from build123d import *

# Parameters (mm, degrees)
F0_R     = 1.651
F0_W     = 83.9253333333
F0_H     = 2.54
F0_W_2   = 0.7576921484
F0_H_2   = 0.9999891111
F1_DEPTH = 25.4


with BuildPart() as f1:
    # F0 (on Top) → F1 (new body)
    with BuildSketch(Plane.XY):
        Polygon((-45.2646666667, -11.43), (-49.8366666667, -11.43), (-49.8366666667, -19.05), (49.8366666667, -19.05), (49.8366666667, -11.43), (45.2646666667, -11.43), (41.9626666667, -11.43), (-41.9626666667, -11.43), align=None)
        with Locations((-47.5506666667, -15.0114614516)):
            Circle(F0_R, mode=Mode.SUBTRACT)
        with Locations((0.0100299507, -15.2482278645)):
            Circle(F0_R, mode=Mode.SUBTRACT)
        with Locations((47.5506666667, -15.0114614516)):
            Circle(F0_R, mode=Mode.SUBTRACT)
        with BuildLine():
            Line((-49.8366666667, -19.05), (-49.8366666667, -11.43))
            Line((-49.8366666667, -11.43), (-49.8366666667, -5.0728137152))
            ThreePointArc((-49.8366666667, -5.0728137152), (-51.4876666667, -3.4218137152), (-49.8366666667, -1.7708137152))
            Line((-49.8366666667, -1.7708137152), (-49.8366666667, 1.778))
            Line((-49.8366666667, 1.778), (-54.9166666667, 1.778))
            Line((-54.9166666667, 1.778), (-54.9166666667, -19.05301027))
            Line((-54.9166666667, -19.05301027), (-49.8366666667, -19.05301027))
            Line((-49.8366666667, -19.05301027), (-49.8366666667, -19.05))
        make_face()
        Polygon((-45.2646666667, -0.9999891111), (-45.2646666667, -11.43), (-41.9626666667, -11.43), (-41.9626666667, -8.89), (-41.9626666667, -0.9999891111), (-44.5069745183, -0.9999891111), align=None)
        with Locations((0, -10.16)):
            Rectangle(F0_W, F0_H)
        with Locations((-44.8858205925, -0.4999945555)):
            Rectangle(F0_W_2, F0_H_2)
        with BuildLine():
            Line((49.8366666667, -11.43), (49.8366666667, -19.05))
            Line((49.8366666667, -19.05), (49.8366666667, -19.05301027))
            Line((49.8366666667, -19.05301027), (54.9166666667, -19.05301027))
            Line((54.9166666667, -19.05301027), (54.9166666667, 1.778))
            Line((54.9166666667, 1.778), (49.8366666667, 1.778))
            Line((49.8366666667, 1.778), (49.8366666667, -1.7708137152))
            ThreePointArc((49.8366666667, -1.7708137152), (51.0040999624, -2.2543804195), (51.4876666667, -3.4218137152))
            ThreePointArc((51.4876666667, -3.4218137152), (51.0040999624, -4.589247011), (49.8366666667, -5.0728137152))
            Line((49.8366666667, -5.0728137152), (49.8366666667, -11.43))
        make_face()
        Polygon((41.9626666667, -8.89), (41.9626666667, -11.43), (45.2646666667, -11.43), (45.2646666667, -0.9999891111), (44.5069745183, -0.9999891111), (41.9626666667, -0.9999891111), align=None)
        Polygon((-45.2646666667, 1.778), (-45.2646666667, 0), (-44.5069745183, 0), (-41.94509238, 0), (-45.2646666667, 3.81), align=None)
        with BuildLine():
            Line((-54.9166666667, 1.778), (-49.8366666667, 1.778))
            Line((-49.8366666667, 1.778), (-45.2646666667, 1.778))
            Line((-45.2646666667, 1.778), (-45.2646666667, 3.81))
            Line((-45.2646666667, 3.81), (-52.8846666667, 3.81))
            ThreePointArc((-52.8846666667, 3.81), (-54.321507646, 3.2148409794), (-54.9166666667, 1.778))
        make_face()
        with Locations((44.8858205925, -0.4999945555)):
            Rectangle(F0_W_2, F0_H_2)
        with BuildLine():
            Line((49.8366666667, 1.778), (54.9166666667, 1.778))
            ThreePointArc((54.9166666667, 1.778), (54.321507646, 3.2148409794), (52.8846666667, 3.81))
            Line((52.8846666667, 3.81), (47.8046666667, 3.81))
            Line((47.8046666667, 3.81), (45.2646666667, 3.81))
            Line((45.2646666667, 3.81), (45.2646666667, 1.778))
            Line((45.2646666667, 1.778), (49.8366666667, 1.778))
        make_face()
        Polygon((44.5069745183, 0), (45.2646666667, 0), (45.2646666667, 1.778), (45.2646666667, 3.81), (41.94509238, 0), align=None)
        with BuildLine():
            Line((-49.8366666667, -5.0728137152), (-49.8366666667, -11.43))
            Line((-49.8366666667, -11.43), (-45.2646666667, -11.43))
            Line((-45.2646666667, -11.43), (-45.2646666667, -0.9999891111))
            Line((-45.2646666667, -0.9999891111), (-45.2646666667, 0))
            Line((-45.2646666667, 0), (-45.2646666667, 1.778))
            Line((-45.2646666667, 1.778), (-49.8366666667, 1.778))
            Line((-49.8366666667, 1.778), (-49.8366666667, -1.7708137152))
            ThreePointArc((-49.8366666667, -1.7708137152), (-48.6692333709, -2.2543804195), (-48.1856666667, -3.4218137152))
            ThreePointArc((-48.1856666667, -3.4218137152), (-48.6692333709, -4.589247011), (-49.8366666667, -5.0728137152))
        make_face()
        with BuildLine():
            Line((45.2646666667, -11.43), (49.8366666667, -11.43))
            Line((49.8366666667, -11.43), (49.8366666667, -5.0728137152))
            ThreePointArc((49.8366666667, -5.0728137152), (48.1856666667, -3.4218137152), (49.8366666667, -1.7708137152))
            Line((49.8366666667, -1.7708137152), (49.8366666667, 1.778))
            Line((49.8366666667, 1.778), (45.2646666667, 1.778))
            Line((45.2646666667, 1.778), (45.2646666667, 0))
            Line((45.2646666667, 0), (45.2646666667, -0.9999891111))
            Line((45.2646666667, -0.9999891111), (45.2646666667, -11.43))
        make_face()
    extrude(amount=F1_DEPTH)


solid = f1.part
The listing builds one solid part. Answer for the finished solid, in the listing's coordinates (mm). A direction names the side the tool comes from. Give positions to 0.01 mm unless a question says otherwise; leave off trailing zeros. Write each loop counter-clockwise with the first axis right and the second up, starting at its lowest first coordinate (ties: lowest second). Pieces come first, ordered by that corner, then holes.
1) A tool of negligible diameter and unlimited length cuts with its end or side. For faces 4 (the face through (-43, -1, 13)), 5 (the face through (-1, -8.89, 13)), 6 (the face through (49, 3.81, 13)), from which of +Z, -Z, +X, -X, +Y, -Y can it reach the whole face along a straight path? Write none if from no direction.
2) Section B-B (x = -37) is taken. Write down the section's boundary in (y, z), and give its area (3 significant figures).
3) Find the intervals of material crossed by L1, parallel to X at y = -0.25, z = 12.5; L2, parallel to X at y = -15, z = 14.75; L3, parallel to Y at x = -50, z = 21, in increasing order.
4) Section A-A (z = 23.75) is taken. Count the separate pieces of the cut face and the enclosed holes in it, and give its area (3 significant figures).
5) For a pull along Y with two mould halves and no side action, classify faces 1 (the face through (54.917, -9, 13)), 2 (the face through (54.337, 3.199, 12.522)), 3 (the face through (43, 0, 13)) as pulls with the +Y half, pulls with the -Y half, needs draft (parallel to the pull), parting line crosses it, or undercut.
6) Given P1, Ø0.8, axis at x = -43.5, z = 12, coming from the -Y side; P2, Ø12.5, axis at x = 10, z = 16.5, coming from the +Y side; P3, Ø2, axis at x = -43.5, z = 17.5, coming from the +Y side, each flat-ended and moving along its own axis, determine where each tip first touches the part or whether it passes through.
Response:
1. face 4: +Z, -Z
1. face 5: +Z, -Z, +Y
1. face 6: +Z, -Z, +X, -X, +Y
2. outline: (-19.05, 0) - (-8.89, 0) - (-8.89, 25.4) - (-19.05, 25.4) - close
2. area: 258 mm2
3. L1: x = -54.92 to -44.51, 44.51 to 54.92
3. L2: x = -54.92 to -49.2, -45.9 to -1.62, 1.64 to 45.9, 49.2 to 54.92
3. L3: y = -19.05 to -5.06, -1.78 to 3.81
4. separate pieces: 1
4. enclosed holes: 5
4. area: 1,380 mm2
5. face 1: needs draft
5. face 2: pulls with the +Y half
5. face 3: undercut
6. P1: stops at y = -19.05
6. P2: stops at y = -8.89
6. P3: stops at y = 2.93
